```python
from build123d import *

# Parameters (mm, degrees)
BOSS_EXTRUDE1_DEPTH = 2.5
FILLET1_R           = 5
SKETCH2_W           = 96.44
SKETCH2_H           = 57
SKETCH2_W_2         = 92.44
SKETCH2_H_2         = 53
BOSS_EXTRUDE2_DEPTH = 85
SKETCH4_W           = 92.44
SKETCH4_H           = 53
CUT_EXTRUDE1_DEPTH  = 104.813534763
SKETCH3_W           = 96.44
SKETCH3_H           = 57
BOSS_EXTRUDE3_DEPTH = 2
BOSS_EXTRUDE4_DEPTH = 96.44
SKETCH6_W           = 5
SKETCH6_H           = 5
BOSS_EXTRUDE5_DEPTH = 85
SKETCH7_R           = 1.6
CUT_EXTRUDE2_DEPTH  = 106.870203551
SKETCH8_W           = 25
SKETCH8_H           = 10
CUT_EXTRUDE3_DEPTH  = 136.694798721
SKETCH9_R           = 1.5
SKETCH9_R_2         = 1.08347565
SKETCH9_R_3         = 1.156670199
CUT_EXTRUDE4_DEPTH  = 106.457337345


with BuildPart() as part:
    # Sketch1 → Boss-Extrude1 (new body)
    with BuildSketch(Plane(origin=(0, 0, 0), x_dir=(1, 0, 0), z_dir=(0, 1, 0))):
        with BuildLine():
            Line((-46.5, 30), (46.5, 30))
            ThreePointArc((46.5, 30), (50.035533906, 28.535533906), (51.5, 25))
            Line((51.5, 25), (51.5, -25))
            ThreePointArc((51.5, -25), (50.035533906, -28.535533906), (46.5, -30))
            Line((46.5, -30), (-46.5, -30))
            ThreePointArc((-46.5, -30), (-50.035533906, -28.535533906), (-51.5, -25))
            Line((-51.5, -25), (-51.5, 25))
            ThreePointArc((-51.5, 25), (-50.035533906, 28.535533906), (-46.5, 30))
        make_face()
    extrude(amount=BOSS_EXTRUDE1_DEPTH)

    # Fillet1
    # the kernel refuses this fillet: 5 mm, written as the material it takes off along each edge
    with BuildSketch(Plane(origin=(-46.5, 2.5, -25), x_dir=(-1, 0, 0), z_dir=(0, 0, 1))) as fillet1_piece_1:
        with BuildLine():
            CenterArc((0.669872981, 5), FILLET1_R, 270, 60)
            Line((0.669872981, 0), (0.669872981, -0.1))
            Line((0.669872981, -0.1), (5, -0.1))
            Line((5, -0.1), (5.1, 0))
            ThreePointArc((5.1, 0), (5.1, 1.25), (5.08660254, 2.45))
            Line((5.08660254, 2.45), (5, 2.5))
        make_face()
    revolve(axis=Axis((-46.5, 2.5, -25), (0, -1, 0)), revolution_arc=90, mode=Mode.SUBTRACT)
    with BuildSketch(Plane(origin=(-46.5, 2.5, -30), x_dir=(0, -1, 0), z_dir=(1, 0, 0)), Plane(origin=(46.5, 2.5, 30), x_dir=(0, -1, 0), z_dir=(-1, 0, 0))) as fillet1_piece_2:
        with BuildLine():
            CenterArc((5, -4.330127019), FILLET1_R, 120, 60)
            Line((0, -4.330127019), (-0.1, -4.330127019))
            Line((-0.1, -4.330127019), (-0.1, 0))
            Line((-0.1, 0), (0, 0.1))
            ThreePointArc((0, 0.1), (1.25, 0.1), (2.45, 0.08660254))
            Line((2.45, 0.08660254), (2.5, 0))
        make_face()
    extrude(amount=93, mode=Mode.SUBTRACT)
    with BuildSketch(Plane(origin=(46.5, 2.5, -25), x_dir=(0, 0, -1), z_dir=(-1, 0, 0))) as fillet1_piece_3:
        with BuildLine():
            CenterArc((0.669872981, 5), FILLET1_R, 270, 60)
            Line((0.669872981, 0), (0.669872981, -0.1))
            Line((0.669872981, -0.1), (5, -0.1))
            Line((5, -0.1), (5.1, 0))
            ThreePointArc((5.1, 0), (5.1, 1.25), (5.08660254, 2.45))
            Line((5.08660254, 2.45), (5, 2.5))
        make_face()
    revolve(axis=Axis((46.5, 2.5, -25), (0, -1, 0)), revolution_arc=90, mode=Mode.SUBTRACT)
    with BuildSketch(Plane(origin=(51.5, 2.5, -25), x_dir=(0, -1, 0), z_dir=(0, 0, 1)), Plane(origin=(-51.5, 2.5, 25), x_dir=(0, -1, 0), z_dir=(0, 0, -1))) as fillet1_piece_4:
        with BuildLine():
            CenterArc((5, -4.330127019), FILLET1_R, 120, 60)
            Line((0, -4.330127019), (-0.1, -4.330127019))
            Line((-0.1, -4.330127019), (-0.1, 0))
            Line((-0.1, 0), (0, 0.1))
            ThreePointArc((0, 0.1), (1.25, 0.1), (2.45, 0.08660254))
            Line((2.45, 0.08660254), (2.5, 0))
        make_face()
    extrude(amount=50, mode=Mode.SUBTRACT)
    with BuildSketch(Plane(origin=(46.5, 2.5, 25), x_dir=(1, 0, 0), z_dir=(0, 0, -1))) as fillet1_piece_5:
        with BuildLine():
            CenterArc((0.669872981, 5), FILLET1_R, 270, 60)
            Line((0.669872981, 0), (0.669872981, -0.1))
            Line((0.669872981, -0.1), (5, -0.1))
            Line((5, -0.1), (5.1, 0))
            ThreePointArc((5.1, 0), (5.1, 1.25), (5.08660254, 2.45))
            Line((5.08660254, 2.45), (5, 2.5))
        make_face()
    revolve(axis=Axis((46.5, 2.5, 25), (0, -1, 0)), revolution_arc=90, mode=Mode.SUBTRACT)
    with BuildSketch(Plane(origin=(-46.5, 2.5, 25), x_dir=(0, 0, 1), z_dir=(1, 0, 0))) as fillet1_piece_6:
        with BuildLine():
            CenterArc((0.669872981, 5), FILLET1_R, 270, 60)
            Line((0.669872981, 0), (0.669872981, -0.1))
            Line((0.669872981, -0.1), (5, -0.1))
            Line((5, -0.1), (5.1, 0))
            ThreePointArc((5.1, 0), (5.1, 1.25), (5.08660254, 2.45))
            Line((5.08660254, 2.45), (5, 2.5))
        make_face()
    revolve(axis=Axis((-46.5, 2.5, 25), (0, -1, 0)), revolution_arc=90, mode=Mode.SUBTRACT)

    # Sketch2 → Boss-Extrude2 (add)
    with BuildSketch(Plane.XZ):
        Rectangle(SKETCH2_W, SKETCH2_H)
        Rectangle(SKETCH2_W_2, SKETCH2_H_2, mode=Mode.SUBTRACT)
    extrude(amount=BOSS_EXTRUDE2_DEPTH)

    # Sketch4 → Cut-Extrude1 (cut, through all)
    with BuildSketch(Plane.XZ):
        Rectangle(SKETCH4_W, SKETCH4_H)
    extrude(amount=-CUT_EXTRUDE1_DEPTH, mode=Mode.SUBTRACT)

    # Sketch3 → Boss-Extrude3 (add)
    with BuildSketch(Plane.XZ.offset(85)):
        Rectangle(SKETCH3_W, SKETCH3_H)
    extrude(amount=BOSS_EXTRUDE3_DEPTH)

    # Sketch5 → Boss-Extrude4 (add)
    with BuildSketch(Plane.ZY.offset(48.22)):
        Polygon((-28.5, -7.5), (-28.5, -3), (-30, -4.114730389), align=None)
    boss_extrude4 = extrude(amount=-BOSS_EXTRUDE4_DEPTH)

    # Mirror1: Boss-Extrude4 across plane
    add(boss_extrude4.mirror(Plane.XY))

    # Sketch6 → Boss-Extrude5 (add)
    with BuildSketch(Plane(origin=(0, -85, 0), x_dir=(1, 0, 0), z_dir=(0, 1, 0))):
        with Locations((43.72, 24)):
            Rectangle(SKETCH6_W, SKETCH6_H)
        with Locations((-43.72, 24)):
            Rectangle(SKETCH6_W, SKETCH6_H)
        with Locations((43.72, -24)):
            Rectangle(SKETCH6_W, SKETCH6_H)
        with Locations((-43.72, -24)):
            Rectangle(SKETCH6_W, SKETCH6_H)
    extrude(amount=BOSS_EXTRUDE5_DEPTH)

    # Sketch7 → Cut-Extrude2 (cut, through all)
    with BuildSketch(Plane(origin=(0, -85, 0), x_dir=(1, 0, 0), z_dir=(0, 1, 0))):
        with Locations(Location((-38.5, 16.5, 0), (0, 0, 270))):
            Circle(SKETCH7_R)
        with Locations(Location((38.5, 16.5, 0), (0, 0, 270))):
            Circle(SKETCH7_R)
        with Locations(Location((-38.5, -16.5, 0), (0, 0, 270))):
            Circle(SKETCH7_R)
        with Locations(Location((38.5, -16.5, 0), (0, 0, 270))):
            Circle(SKETCH7_R)
    extrude(amount=-CUT_EXTRUDE2_DEPTH, mode=Mode.SUBTRACT)

    # Sketch8 → Cut-Extrude3 (cut, through all)
    with BuildSketch(Plane(origin=(48.22, 0, 0), x_dir=(0, 0, -1), z_dir=(1, 0, 0))):
        with Locations((-3.355310765, -74.801411427)):
            Rectangle(SKETCH8_W, SKETCH8_H)
    extrude(amount=-CUT_EXTRUDE3_DEPTH, mode=Mode.SUBTRACT)

    # Sketch9 → Cut-Extrude4 (cut, through all)
    with BuildSketch(Plane(origin=(0, 0, 0), x_dir=(1, 0, 0), z_dir=(0, 1, 0))):
        with Locations(Location((-43.72, -24, 0), (0, 0, 270))):
            Circle(SKETCH9_R)
        with Locations(Location((43.72, -24, 0), (0, 0, 270))):
            Circle(SKETCH9_R)
        with Locations(Location((43.72, 24, 0), (0, 0, 270))):
            Circle(SKETCH9_R_2)
        with Locations(Location((-43.72, 24, 0), (0, 0, 270))):
            Circle(SKETCH9_R_3)
    extrude(amount=-CUT_EXTRUDE4_DEPTH, mode=Mode.SUBTRACT)


solid = part.part
```
Model file for the job. Use its own axes, mm. A direction names the side the tool comes from. Coordinates: 2 decimals unless noted, no trailing zeros. Loops run counter-clockwise (first coordinate to the right, second up) from the corner with the lowest first, then second, coordinate; pieces in that order, holes last. Notation, with made-up numbers: (78, 65) - (110, 65) arc R3 ccw to (110, 70) - close; hole circle Ø11 at (-32, 21.5). An arc over 180 degrees is marked (long way). Write item = value, one per line. Start each with the question number.
Item 1: Drop flat-ended pins along their axis: pin 1 Ø1.5 at (x, z) = (29.5, 14.5) entering from +Y; pin 2 Ø2.5 at (x, z) = (-43.5, -25) entering from +Y; pin 3 Ø2 at (x, y) = (-47, -72.5) entering from -Z. Give the stop position or say it passes through.
Item 2: Pull direction X, two halves, no side cores. Call faces 1 (the face through (42, 0, 24)), 2 (the face through (-1, -47, 28.5)), 3 (the face through (-41.22, -43, -24)), 4 (the face through (49.702, 1.812, -0.35)): +X half, -X half, draft (parallel to the pull), parting line (faces both ways), or undercut.
Item 3: Saw through at B-B, the plane x = -38.5. List the corners of the cut face in (y, z), then the cut area to 3 significant figures.
Item 4: Saw through at C-C, the plane y = -71. List the corners of the cut face in (x, z).
Item 5: Wall check: probe 1 along Z at (x, y) = (-28.5, -70); probe 2 along X at (y, z) = (-42, 0); probe 3 along Y at (x, z) = (-26.5, 12). Give the ranges that are in metal, low to high. Write a range as [from, to].
Item 6: Saw through at A-A, the plane z = -16.5. List the corners of the cut face in (x, y).
Item 7: 3-axis set-ups, long thin cutter, end or side, ignore diameter. For faces 5 (the face through (48.22, -43, 0)), 6 (the face through (-1, -1, 28.5)), 7 (the face through (44, -43, -21.5)), 8 (the face through (-0.68, -5.78, -29.26)): which of +Z, -Z, +X, -X, +Y, -Y reach the whole face in a straight line?
Item 8: Saw through at D-D, the plane x = -11.5. List the corners of the cut face in (y, z).
Answers:
q1.pin_1 = -85
q1.pin_2 = 0
q1.pin_3 = -28.5
q2.face_1 = undercut
q2.face_2 = draft
q2.face_3 = undercut
q2.face_4 = +X half
q3.outline = (-87, -28.5) - (-7.5, -28.5) - (-4.11, -30) - (-3, -28.5) - (0, -28.5) - (0, -30) arc R5 ccw to (2.43, -26.5) - (-85, -26.5) - (-85, -18.1) - (-87, -18.1) - close; (-87, -14.9) - (-85, -14.9) - (-85, 14.9) - (-87, 14.9) - close; (-87, 18.1) - (-85, 18.1) - (-85, 26.5) - (2.43, 26.5) arc R5 ccw to (0, 30) - (0, 28.5) - (-3, 28.5) - (-4.11, 30) - (-7.5, 28.5) - (-87, 28.5) - close
q3.area = 459 mm2
q4.outline = (-48.22, -28.5) - (48.22, -28.5) - (48.22, -9.14) - (46.22, -9.14) - (46.22, -21.5) - (41.22, -21.5) - (41.22, -26.5) - (-41.22, -26.5) - (-41.22, -21.5) - (-46.22, -21.5) - (-46.22, -9.14) - (-48.22, -9.14) - close; (-48.22, 15.86) - (-46.22, 15.86) - (-46.22, 21.5) - (-41.22, 21.5) - (-41.22, 26.5) - (41.22, 26.5) - (41.22, 21.5) - (46.22, 21.5) - (46.22, 15.86) - (48.22, 15.86) - (48.22, 28.5) - (-48.22, 28.5) - close; hole circle Ø3 at (-43.72, 24); hole circle Ø2.31 at (-43.72, -24); hole circle Ø3 at (43.72, 24); hole circle Ø2.17 at (43.72, -24)
q5.probe_1 = [-28.5, -26.5], [26.5, 28.5]
q5.probe_2 = [-48.22, -46.22], [46.22, 48.22]
q5.probe_3 = [-87, -85]
q6.outline = (-51.5, 0) - (-48.22, 0) - (-48.22, -87) - (-40.1, -87) - (-40.1, -85) - (-46.22, -85) - (-46.22, 2.5) - (-47.17, 2.5) arc R5 ccw to start; (-36.9, -87) - (36.9, -87) - (36.9, -85) - (-36.9, -85) - close; (40.1, -87) - (48.22, -87) - (48.22, 0) - (51.5, 0) arc R5 ccw to (47.17, 2.5) - (46.22, 2.5) - (46.22, -85) - (40.1, -85) - close
q7.face_5 = +Z, -Z, +X, -Y
q7.face_6 = +Z, +X, -X
q7.face_7 = +Y
q7.face_8 = -Z, +X, -X, -Y
q8.outline = (-87, -28.5) - (-7.5, -28.5) - (-4.11, -30) - (-3, -28.5) - (0, -28.5) - (0, -30) arc R5 ccw to (2.43, -26.5) - (-85, -26.5) - (-85, 26.5) - (2.43, 26.5) arc R5 ccw to (0, 30) - (0, 28.5) - (-3, 28.5) - (-4.11, 30) - (-7.5, 28.5) - (-87, 28.5) - close
